The listing builds one solid part. Answer for the finished solid, in the listing's coordinates (mm). A direction names the side the tool comes from. Coordinates: 2 decimals unless noted, no trailing zeros. Loops run counter-clockwise (first coordinate to the right, second up) from the corner with the lowest first, then second, coordinate; pieces in that order, holes last. Notation, with made-up numbers: M -39.75,60.25 L -34.75,60.25 A11 ccw -34.75,80.25 Z; hole C 17,57 d2. An arc over 180 degrees is marked long. Return JSON: item names as keys, results as strings. Group by question number.
1. Section A-A (x = 13) is taken. Write down the section's boundary in (y, z).
2. Straight lines are drawn through the part: L1, parallel to Y at x = 3.25, z = 0; L2, parallel to Z at x = -17.5, y = 0. For each, find the intervals that lie inside material, in ascending order. Write a range as from..to.
3. Section C-C (z = -39) is taken. Write down the section's boundary in (x, y), then the cut area to 3 significant figures.
4. Which of the six approach directions +Z, -Z, +X, -X, +Y, -Y give full straight-line access (tool end or side, diameter ignored) to faces 1 (the face through (22.686, 17.4, -17.5)), 2 (the face through (15.784, 22.226, 9.056)), 3 (the face through (15.78, 22.12, -9.31)), 4 (the face through (15.78, -22.12, 9.31)), 5 (the face through (-18.314, 14, -32))?
5. Section B-B (x = -16.5) is taken. Write down the section's boundary in (y, z), then the cut area to 3 significant figures.
6. The mould has two halves that part along Z. Classify faces 6 (the face through (22.686, 25, 0)), 7 (the face through (30.826, 4.802, 21.623)), 8 (the face through (15.784, -9.056, 22.226)): pulls with the +Z half, pulls with the -Z half, needs draft (parallel to the pull), parting line crosses it, or undercut.
7. Given P1, Ø1, axis at y = 21.5, z = -10.5, coming from the -X side; P2, Ø5, axis at y = 24.5, z = -24.5, coming from the +X side; P3, Ø0.8, axis at y = -25.5, z = -2, coming from the +X side; P4, Ø6, axis at x = 30.5, z = 29, coming from the +Y side, each flat-ended and moving along its own axis, determine where each tip first touches the part or whether it passes through.
```python
from build123d import *

# Parameters (mm, degrees)
CUT_EXTRUDE1_START = -27
SKETCH2_R          = 61.415464326
CUT_EXTRUDE1_DEPTH = 27
SKETCH3_R          = 40.122085913
CUT_EXTRUDE2_DEPTH = 14


with BuildPart() as part:
    # Sketch1 → Revolve1 (revolve)
    with BuildSketch(Plane.XY):
        Polygon((-32.314138911, -25), (-8.814138911, -25), (-8.814138911, -17), (20.685861089, -17), (20.685861089, -22.15), (40.685861089, -22.15), (40.685861089, -23.757238603), (22.685861089, -24.15), (22.685861089, -34.74048531), (8.685861089, -34.74048531), (8.685861089, -47.75), (-18.314138911, -47.75), (-18.314138911, -34), (-32.314138911, -34), align=None)
    revolve(axis=Axis((0, 0, 0), (1, 0, 0)))

    # Sketch2 → Cut-Extrude1 (cut)
    with BuildSketch(Plane(origin=(8.685861089, 0, 0), x_dir=(0, 0, -1), z_dir=(1, 0, 0)).offset(CUT_EXTRUDE1_START)):
        Circle(SKETCH2_R)
        Polygon((0, 48.707649013), (-34.441508913, 34.441508913), (-48.707649013, 0), (-34.441508913, -34.441508913), (0, -48.707649013), (34.441508913, -34.441508913), (48.707649013, 0), (34.441508913, 34.441508913), align=None, mode=Mode.SUBTRACT)
    extrude(amount=CUT_EXTRUDE1_DEPTH, mode=Mode.SUBTRACT)

    # Sketch3 → Cut-Extrude2 (cut)
    with BuildSketch(Plane(origin=(22.685861089, 0, 0), x_dir=(0, 0, -1), z_dir=(1, 0, 0))):
        Circle(SKETCH3_R)
        Polygon((0, 25.977412807), (-18.368804754, 18.368804754), (-25.977412807, 0), (-18.368804754, -18.368804754), (0, -25.977412807), (18.368804754, -18.368804754), (25.977412807, 0), (18.368804754, 18.368804754), align=None, mode=Mode.SUBTRACT)
    extrude(amount=-CUT_EXTRUDE2_DEPTH, mode=Mode.SUBTRACT)


solid = part.part
```
Worked out:
{
 "1": {"outline": "M -25.98,0 L -18.37,-18.37 L 0,-25.98 L 18.37,-18.37 L 25.98,0 L 18.37,18.37 L 0,25.98 L -18.37,18.37 Z; hole C 0,0 d34"},
 "2": {"L1": "-47.75..-17, 17..47.75", "L2": "-47.75..-25, 25..47.75"},
 "3": {"outline": "M -18.31,-23.44 L 8.69,-23.44 L 8.69,23.44 L -18.31,23.44 Z", "area": "1,270 mm^2"},
 "4": {"face 1": "-Z, +X, +Y", "face 2": "+Z, +Y", "face 3": "-Z, +Y", "face 4": "+Z, -Y", "face 5": "-X"},
 "5": {"outline": "M -47.69,-2.47 L -35.46,-31.98 A47.75 ccw -31.98,-35.46 L -2.47,-47.69 A47.75 ccw 2.47,-47.69 L 31.98,-35.46 A47.75 ccw 35.46,-31.98 L 47.69,-2.47 A47.75 ccw 47.69,2.47 L 35.46,31.98 A47.75 ccw 31.98,35.46 L 2.47,47.69 A47.75 ccw -2.47,47.69 L -31.98,35.46 A47.75 ccw -35.46,31.98 L -47.69,2.47 A47.75 ccw Z; hole C 0,0 d50", "area": "4,730 mm^2"},
 "6": {"face 6": "needs draft", "face 7": "undercut", "face 8": "pulls with the +Z half"},
 "7": {"P1": "x = -8.81", "P2": "x = 8.69", "P3": "x = 22.69", "P4": "through"}
}
